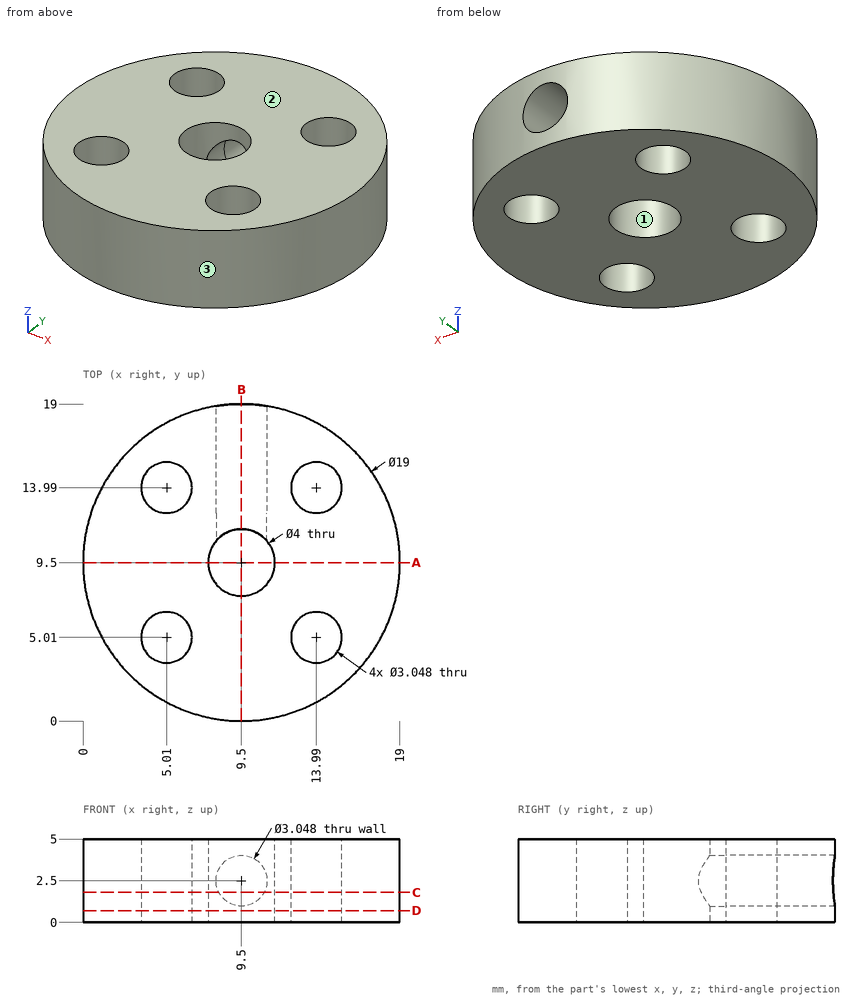
Design review of the part shown in the three views and the two pictorial views. Dimensions are in mm from the part's minimum x, y and z. Give positions to 0.01 mm unless a question says otherwise; leave off trailing zeros. Write each loop counter-clockwise with the first axis right and the second up, starting at its lowest first coordinate (ties: lowest second). Pieces come first, ordered by that corner, then holes.
Item 1: The part is to be moulded in two halves that separate along X. For the marked faces 1, 2 and 3, say which applies: +X half, -X half, draft (parallel to the pull), parting line (faces both ways), or undercut.
Item 2: Wall thickness on probe 1 along Y at (x, z) = (4, 3.5); probe 2 along X at (y, z) = (14.5, 2.4); probe 3 along Y at (x, z) = (4.5, 4.05): over which ranges is each line inside the solid? List them lowest first.
Item 3: Take a section at A-A (y = 9.5). Give the boundary of the cut face in (x, z).
Item 4: Insertion check: P1, Ø2.5, axis at x = 9.5, z = 2.5, coming from the +Y side; P2, Ø1, axis at y = 4, z = 2, coming from the -X side; P3, Ø1.5, axis at x = 13, z = 4.5, coming from the +Y side. Each pin has a flat end and moves straight along its axis. Give the tip position at first contact, or say it passes through.
Item 5: Take a section at C-C (z = 1.8). Give the boundary of the cut face in (x, y).
Item 6: Take a section at D-D (z = 0.7). Give the boundary of the cut face in (x, y).
Item 7: Take a section at B-B (x = 9.5). Give the boundary of the cut face in (y, z).
Established:
1. face 1: undercut
1. face 2: draft
1. face 3: parting line
2. probe 1: y = 1.75 to 3.87, 6.15 to 12.85, 15.13 to 17.25
2. probe 2: x = 1.42 to 3.57, 6.45 to 7.98, 11.02 to 12.55, 15.43 to 17.58
2. probe 3: y = 1.42 to 3.57, 6.45 to 12.55, 15.43 to 17.58
3. outline: (0, 0) - (7.5, 0) - (7.5, 5) - (0, 5) - close; (11.5, 0) - (19, 0) - (19, 5) - (11.5, 5) - close
4. P1: stops at y = 7.94
4. P2: stops at x = 1.42
4. P3: stops at y = 18.59
5. outline: (8.15, 10.97) - (8.15, 18.9) arc R9.5 ccw (long way) to (10.85, 18.9) - (10.85, 10.97) arc R2 cw (long way) to start; hole circle Ø3.05 at (5.01, 5.01); hole circle Ø3.05 at (5.01, 13.99); hole circle Ø3.05 at (13.99, 5.01); hole circle Ø3.05 at (13.99, 13.99)
6. outline: circle Ø19 at (9.5, 9.5); hole circle Ø3.05 at (5.01, 5.01); hole circle Ø3.05 at (5.01, 13.99); hole circle Ø4 at (9.5, 9.5); hole circle Ø3.05 at (13.99, 5.01); hole circle Ø3.05 at (13.99, 13.99)
7. outline: (0, 0) - (7.5, 0) - (7.5, 5) - (0, 5) - close; (11.5, 0) - (19, 0) - (19, 0.98) - (11.5, 0.98) - close; (11.5, 4.02) - (19, 4.02) - (19, 5) - (11.5, 5) - close
